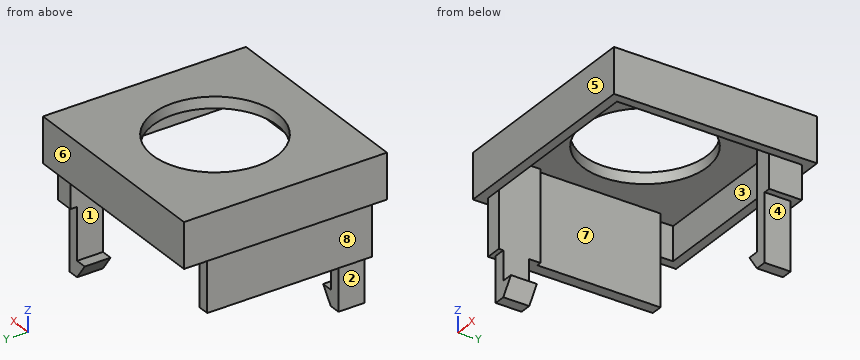
from build123d import *

# Parameters (mm, degrees)
SKETCH045_W     = 18.5
SKETCH045_H     = 18
PAD029_DEPTH    = 4
SKETCH046_W     = 16.9
SKETCH046_H     = 16.4
POCKET014_DEPTH = 3
SKETCH047_R     = 5.5
POCKET015_DEPTH = 5
SKETCH048_W     = 1
SKETCH048_H     = 2.3
PAD030_DEPTH    = 12
SKETCH049_W     = 1
SKETCH049_H     = 2.3
PAD031_DEPTH    = 1.4
POCKET016_DEPTH = 2.3
POCKET017_DEPTH = 2.3
PAD071_DEPTH    = 8
SKETCH133_W     = 1.6
SKETCH133_H     = 2.9
PAD072_DEPTH    = 6


with BuildPart() as part:
    # Sketch045 → Pad029 (new body)
    with BuildSketch(Plane(origin=(78.2, -39.95, 23), x_dir=(1, 0, 0), z_dir=(0, 0, 1))):
        Rectangle(SKETCH045_W, SKETCH045_H)
    extrude(amount=PAD029_DEPTH)

    # Sketch046 (on Face5 of Pad029) → Pocket014 (cut)
    with BuildSketch(Plane(origin=(0, 0, 23), x_dir=(1, 0, 0), z_dir=(0, 0, -1))):
        with Locations((78.2, 39.95)):
            Rectangle(SKETCH046_W, SKETCH046_H)
    extrude(amount=-POCKET014_DEPTH, mode=Mode.SUBTRACT)

    # Sketch047 (on Face5 of Pocket014) → Pocket015 (cut)
    with BuildSketch(Plane.XY.offset(27)):
        with Locations((78.2, -39.95)):
            Circle(SKETCH047_R)
    extrude(amount=-POCKET015_DEPTH, mode=Mode.SUBTRACT)

    # Sketch048 (on Face12 of Pocket015) → Pad030 (join)
    with BuildSketch(Plane(origin=(0, 0, 26), x_dir=(1, 0, 0), z_dir=(0, 0, -1))):
        with Locations((85.55, 33.5)):
            Rectangle(SKETCH048_W, SKETCH048_H)
        with Locations((70.65, 46.6)):
            Rectangle(SKETCH048_W, SKETCH048_H)
    extrude(amount=PAD030_DEPTH)

    # Sketch049 (on Face21 of Pad030) → Pad031 (join)
    with BuildSketch(Plane(origin=(0, 0, 14), x_dir=(1, 0, 0), z_dir=(0, 0, -1))):
        with Locations((71.65, 46.6)):
            Rectangle(SKETCH049_W, SKETCH049_H)
        with Locations((84.55, 33.5)):
            Rectangle(SKETCH049_W, SKETCH049_H)
    extrude(amount=-PAD031_DEPTH)

    # Sketch050 (on Face24 of Pad031) → Pocket016 (cut)
    with BuildSketch(Plane(origin=(0, -45.45, 0), x_dir=(-1, 0, 0), z_dir=(0, 1, 0))):
        Polygon((-72.15, 15.4), (-71.15, 14), (-72.15, 14), align=None)
    extrude(amount=-POCKET016_DEPTH, mode=Mode.SUBTRACT)

    # Sketch051 (on Face28 of Pocket016) → Pocket017 (cut)
    with BuildSketch(Plane.XZ.offset(34.65)):
        Polygon((85.05, 14), (84.05, 15.4), (84.05, 14), align=None)
    extrude(amount=-POCKET017_DEPTH, mode=Mode.SUBTRACT)

    # Sketch132 (on Face12 of Pocket017) → Pad071 (join)
    with BuildSketch(Plane(origin=(0, 0, 26), x_dir=(1, 0, 0), z_dir=(0, 0, -1))):
        Polygon((71.15, 48.15), (69.75, 48.15), (69.75, 33.55), (70.75, 33.55), (70.75, 44.45), (71.15, 44.45), align=None)
    extrude(amount=PAD071_DEPTH)

    # Sketch133 (on Face18 of Pad071) → Pad072 (join)
    with BuildSketch(Plane(origin=(0, 0, 26), x_dir=(1, 0, 0), z_dir=(0, 0, -1))):
        with Locations((85.85, 33.2)):
            Rectangle(SKETCH133_W, SKETCH133_H)
    extrude(amount=PAD072_DEPTH)


with BuildPart() as part_1:
    # Body015 placement: moved
    add(part.part.moved(Location((0, 0, -4))))


solid = part_1.part
Part model, mm, in its own coordinate system. Face numbers are marked on the shaded views. A direction names the side the tool comes from. Give positions to 0.01 mm unless a question says otherwise; leave off trailing zeros. Loops run counter-clockwise (first coordinate to the right, second up) from the corner with the lowest first, then second, coordinate; pieces in that order, holes last.
(1) 3-axis set-ups, long thin cutter, end or side, ignore diameter. For the marked faces 1, 2, 3 and 4: which of +Z, -Z, +X, -X, +Y, -Y reach the whole face in a straight line?
Return value:
face 1: none
face 2: -Z, -X, +Y, -Y
face 3: -Z
face 4: -Z, +X, +Y, -Y
(2) Pin check, flat tips, straight feed: pin 1 (5 mm diameter, centred on x = 72.5, y = -40, fed in from -Z); pin 2 (5 mm diameter, centred on x = 74.5, y = -44, fed in from -Z); pin 3 (0.9 mm diameter, centred on y = -32.5, z = 17, fed in from +X). Stop position of each tip, or through.
Return value:
pin 1: stops at z = 14
pin 2: stops at z = 22
pin 3: stops at x = 86.65
(3) Band-saw the part on D-D (z = 18.75). Write the cut outline in (x, y), and give its area (3 significant figures).
Return value:
outline: (69.75, -48.15) - (71.15, -48.15) - (71.15, -44.45) - (70.75, -44.45) - (70.75, -33.55) - (69.75, -33.55) - close; (85.05, -34.65) - (86.65, -34.65) - (86.65, -31.75) - (85.05, -31.75) - close
area: 20.7 mm2
(4) Drill centre lines: line 1 along Y through (x, z) = (78.2, 22.4); line 2 along X through (y, z) = (-45, 21.5); line 3 along Y through (x, z) = (77, 21.5). Where is each one in solid material? Low to high.
Return value:
line 1: y = -48.95 to -45.45, -34.45 to -30.95
line 2: x = 68.95 to 71.15, 86.65 to 87.45
line 3: y = -48.95 to -48.15, -31.75 to -30.95
(5) Pull direction Y, two halves, no side cores. Call the marked faces 5, 6, 7 and 8: pulls with the +Y half, pulls with the -Y half, needs draft (parallel to the pull), parting line crosses it, or undercut.
Return value:
face 5: pulls with the -Y half
face 6: pulls with the +Y half
face 7: undercut
face 8: needs draft
(6) Band-saw the part on C-C (y = -39.95). Write the cut outline in (x, z).
Return value:
outline: (68.95, 19) - (69.75, 19) - (69.75, 14) - (70.75, 14) - (70.75, 22) - (72.7, 22) - (72.7, 23) - (68.95, 23) - close; (83.7, 22) - (86.65, 22) - (86.65, 19) - (87.45, 19) - (87.45, 23) - (83.7, 23) - close
(7) Band-saw the part on B-B (z = 20.25). Write the cut outline in (x, y).
Return value:
outline: (68.95, -48.95) - (87.45, -48.95) - (87.45, -30.95) - (68.95, -30.95) - close; hole (69.75, -33.55) - (70.75, -33.55) - (70.75, -44.45) - (71.15, -44.45) - (71.15, -48.15) - (86.65, -48.15) - (86.65, -34.65) - (85.05, -34.65) - (85.05, -31.75) - (69.75, -31.75) - close
(8) Band-saw the part on A-A (x = 78.2). Write the cut outline in (y, z), and give its area (3 significant figures).
Return value:
outline: (-48.95, 19) - (-48.15, 19) - (-48.15, 22) - (-45.45, 22) - (-45.45, 23) - (-48.95, 23) - close; (-34.45, 22) - (-31.75, 22) - (-31.75, 19) - (-30.95, 19) - (-30.95, 23) - (-34.45, 23) - close
area: 11.8 mm2
